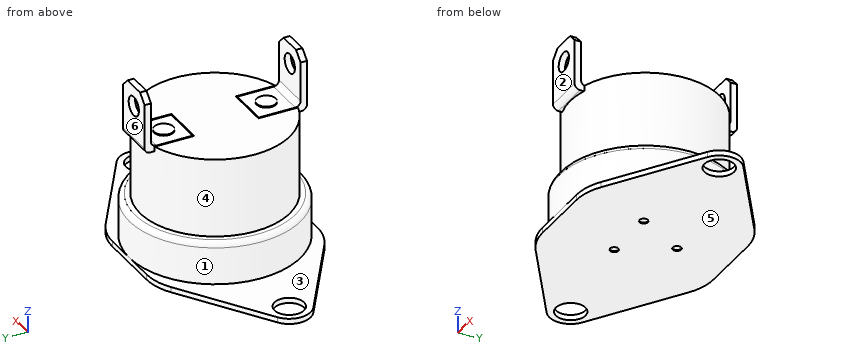
Autodesk Inventor part; units mm, degrees
ref_plane "YZ Plane" through (0, 0, 0) normal (1, 0, 0) x (0, 1, 0)
ref_plane "XZ Plane" through (0, 0, 0) normal (0, 1, 0) x (-1, 0, 0)
ref_plane "XY Plane" through (0, 0, 0) normal (0, 0, 1) x (1, 0, 0)
sketch "Skizze1" plane through (0, 0, 0) normal (0, 0, 1) x (1, 0, 0)
  line L0 (-3, 8) -> (3, 8)
  line L1 (5.7352, 7.1856) -> (14.1691, 1.6742)
  line L2 (14.1691, -1.6742) -> (5.7352, -7.1856)
  line L3 (3, -8) -> (-3, -8)
  line L4 (-5.7352, -7.1856) -> (-14.1691, -1.6742)
  line L5 (-14.1691, 1.6742) -> (-5.7352, 7.1856)
  arc A0 (14.1691, -1.6742) -> (14.1691, 1.6742) centre (13.075, 0) ccw
  arc A1 (-14.1691, 1.6742) -> (-14.1691, -1.6742) centre (-13.075, 0) ccw
  circle A2 centre (0, 0) radius 7
  circle A3 centre (-13.075, 0) radius 1.385
  circle A4 centre (13.075, 0) radius 1.385
  arc A5 (-3, 8) -> (-5.7352, 7.1856) centre (-3, 3) ccw
  arc A6 (5.7352, 7.1856) -> (3, 8) centre (3, 3) ccw
  arc A7 (3, -8) -> (5.7352, -7.1856) centre (3, -3) ccw
  arc A8 (-5.7352, -7.1856) -> (-3, -8) centre (-3, -3) ccw
  dimension "d0" = 16
  dimension "d1" = 8
  dimension "d3" = 2
  dimension "d4" = 14
  dimension "d5" = 30.15
  dimension "d7" = 2.77
  dimension "d8" = 2.77
  dimension "d9" = 13.075
  dimension "d10" = 13.075
  dimension "d11" = 5
  dimension "d12" = 6
  dimension "d13" = 6
  dimension "d14" = 3
  dimension "d15" = 3
extrude "Extrusion1" add sketch "Skizze1" along normal blind 0.5
sketch "Skizze2" plane through (0, 0, 0.5) normal (0, 0, 1) x (1, 0, 0)
  circle A0 centre (0, 0) radius 8
  circle A1 centre (0, 0) radius 7
  dimension "d18" = 16
  dimension "d19" = 14
extrude "Extrusion2" add sketch "Skizze2" along normal blind 4
fillet "Rundung1" radius 0.5 1 edges at (-8, 0, 4.5)
sketch "Skizze3" plane through (0, 0, 0) normal (0, 0, -1) x (-1, 0, 0)
  circle A0 centre (0, 0) radius 7
  dimension "d23" = 14
extrude "Extrusion3" add sketch "Skizze3" against normal blind 11.91
sketch "Skizze4" plane through (0, 0, 0) normal (0, 0, -1) x (-1, 0, 0)
  circle A0 centre (0, 3) radius 0.4
  point P0 (0, 0)
  dimension "d26" = 3
  dimension "d27" = 0.8
extrude "Extrusion4" cut sketch "Skizze4" against normal blind 0.1
pattern_circular "Runde Anordnung1" count 3 over 360 about axis through (0, 0, -10) along (0, 0, 1) of "Extrusion4"
sketch "Skizze5" plane through (0, 0, 11.91) normal (0, 0, 1) x (1, 0, 0)
  line L0 (2, -9) -> (-2, -9)
  line L1 (-2, -9) -> (-2, -3)
  line L2 (-2, -3) -> (2, -3)
  line L3 (2, -3) -> (2, -9)
  line L4 (2, 3) -> (-2, 3)
  line L5 (-2, 3) -> (-2, 9)
  line L6 (-2, 9) -> (2, 9)
  line L7 (2, 9) -> (2, 3)
  line L8 (3, 8) -> (0, 8)
  line L9 (0, -8) -> (3, -8)
  point P0 (0, 0)
  dimension "d33" = 4
  dimension "d34" = 2
  dimension "d35" = 3
  dimension "d36" = 3
  dimension "d37" = 1
  dimension "d38" = 1
extrude "Extrusion5" cut sketch "Skizze5" against normal blind 0.5
sketch "Skizze6" plane through (0, 0, 11.41) normal (0, 0, 1) x (1, 0, 0)
  line L0 (1.9, -7.6) -> (-1.9, -7.6)
  line L1 (-1.9, -7.6) -> (-1.9, -3.1)
  line L2 (-1.9, -3.1) -> (1.9, -3.1)
  line L3 (1.9, -3.1) -> (1.9, -7.6)
  line L4 (-2, -3) -> (2, -3)
  line L5 (1.9, 3.1) -> (-1.9, 3.1)
  line L6 (-1.9, 3.1) -> (-1.9, 7.6)
  line L7 (-1.9, 7.6) -> (1.9, 7.6)
  line L8 (1.9, 7.6) -> (1.9, 3.1)
  line L9 (2, 3) -> (-2, 3)
  point P0 (0, 0)
  dimension "d41" = 3.8
  dimension "d42" = 1.9
  dimension "d43" = 0.1
  dimension "d44" = 4.5
  dimension "d45" = 3.8
  dimension "d46" = 1.9
  dimension "d47" = 0.1
  dimension "d48" = 4.5
extrude "Extrusion6" add sketch "Skizze6" along normal blind 0.5
sketch "Skizze7" plane through (0, 0, 11.91) normal (0, 0, 1) x (1, 0, 0)
  line L0 (1.9, 7.6) -> (-1.9, 7.6)
  line L1 (-1.9, 7.6) -> (-1.9, 3.1)
  line L2 (1.9, 7.6) -> (-1.9, 7.6)
  line L3 (-1.9, 7.6) -> (-1.9, 7)
  line L4 (-1.9, 7) -> (1.9, 7)
  line L5 (1.9, 7) -> (1.9, 7.6)
  line L6 (-1.9, -7.6) -> (1.9, -7.6)
  line L7 (-1.9, -3.1) -> (-1.9, -7.6)
  line L8 (1.9, -7.6) -> (-1.9, -7.6)
  line L9 (-1.9, -7.6) -> (-1.9, -7)
  line L10 (-1.9, -7) -> (1.9, -7)
  line L11 (1.9, -7) -> (1.9, -7.6)
  point P0 (0, 0)
  dimension "d51" = 0.6
  dimension "d52" = 0.6
extrude "Extrusion7" add sketch "Skizze7" along normal blind 5
chamfer "Fase1" distance 0.8 angle 45 4 edges at (-1.9, 7.3, 16.91) (1.9, 7.3, 16.91) (-1.9, -7.3, 16.91) (1.9, -7.3, 16.91)
fillet "Rundung2" radius 0.5 4 edges at (0, 7.6, 11.41) (0, -7.6, 11.41) (0, -7, 11.91) (0, 7, 11.91)
sketch "Skizze8" plane through (-1.1, 7.6, 16.91) normal (0, 1, 0) x (1, 0, 0)
  circle A0 centre (1.1, 1.9) radius 0.9
  line L0 (2.2, 0) -> (0, 0)
  point P0 (1.1, 16.91)
  dimension "d59" = 1.8
  dimension "d60" = 1.9
extrude "Extrusion8" cut sketch "Skizze8" against normal blind 20
sketch "Skizze9" plane through (0, 0, 11.91) normal (0, 0, 1) x (1, 0, 0)
  circle A0 centre (0, 4.8) radius 0.9
  circle A1 centre (0, -4.8) radius 0.9
  point P0 (0, 0)
  dimension "d63" = 1.8
  dimension "d64" = 1.8
  dimension "d65" = 4.8
  dimension "d66" = 4.8
extrude "Extrusion9" add sketch "Skizze9" along normal blind 0.1
properties part number "Bimetallschalter"
Here's how the part is built. I have some questions about the finished solid (model axes, mm). Face numbers are marked on the shaded views. A direction names the side the tool comes from. Round coordinates to 2 decimals unless told otherwise and drop trailing zeros. Loops run counter-clockwise (first coordinate to the right, second up) from the corner with the lowest first, then second, coordinate; pieces in that order, holes last. Notation, with made-up numbers: (83.5, -13.5) -> (100.5, -13.5) arc R25 ccw to (100.5, 1.5) -> close; hole circle Ø7 at (59, 80.25). An arc over 180 degrees is marked (long way). Answer as CSV lines item,"result".
1. If we section it at C-C on z = 9.5: Please give me the cut outline in (x, y).
Final values:
outline,"circle Ø14 at (0, 0)"
2. For pin 1 (1.3 mm diameter, centred on y = -6.5, z = 13, fed in from -X); pin 2 (10 mm diameter, centred on x = -7.5, z = 6, fed in from +Y); pin 3 (5 mm diameter, centred on x = 6, y = 5, fed in from +Z), each with a flat end and sliding along its axis, tell me the tip position at first contact or that it passes through.
Final values:
pin 1,"stops at x = -1.9"
pin 2,"stops at y = 7.46"
pin 3,"stops at z = 11.91"
3. Thinking about a two-plate mould opening in Z: for the marked faces 4, 5 and 6, which applies, released by +Z, released by -Z, zero draft, split by the parting line, or undercut?
Final values:
face 4,"undercut"
face 5,"released by -Z"
face 6,"zero draft"
4. Which directions (+Z, -Z, +X, -X, +Y, -Y) give clear straight access to the entire face, cutting with the end or side of a thin tool? Please do the marked faces 1, 2 and 3.
Final values:
face 1,"+Z"
face 2,"+Z, +X, -X, -Y"
face 3,"+Z, -X"
5. If we section it at B-B on y = 0: Please give me the cut outline in (x, z) (3 decimals).
Final values:
outline,"(-15.075, 0) -> (-14.46, 0) -> (-14.46, 0.5) -> (-15.075, 0.5) -> close; (-11.69, 0) -> (11.69, 0) -> (11.69, 0.5) -> (8, 0.5) -> (8, 4) arc R0.5 ccw to (7.5, 4.5) -> (7, 4.5) -> (7, 11.91) -> (-7, 11.91) -> (-7, 4.5) -> (-7.5, 4.5) arc R0.5 ccw to (-8, 4) -> (-8, 0.5) -> (-11.69, 0.5) -> close; (14.46, 0) -> (15.075, 0) -> (15.075, 0.5) -> (14.46, 0.5) -> close"
6. If we section it at A-A on z = 13.75: Please give me the cut outline in (x, y).
Final values:
outline,"(-1.9, -7.6) -> (1.9, -7.6) -> (1.9, -7) -> (-1.9, -7) -> close; (-1.9, 7) -> (1.9, 7) -> (1.9, 7.6) -> (-1.9, 7.6) -> close"
7. If I drill on L1, parallel to Z at x = 0, y = -7.1; L2, parallel to Y at x = 1, z = 15.5; L3, parallel to X at y = 7.2, z = 15.01, over which ranges is the centre line in solid material (lowest first)?
Final values:
L1,"z = 0 to 4.5, 11.41 to 14.11, 15.91 to 16.91"
L2,"y = -7.6 to -7, 7 to 7.6"
L3,"x = -1.9 to -0.9, 0.9 to 1.9"
